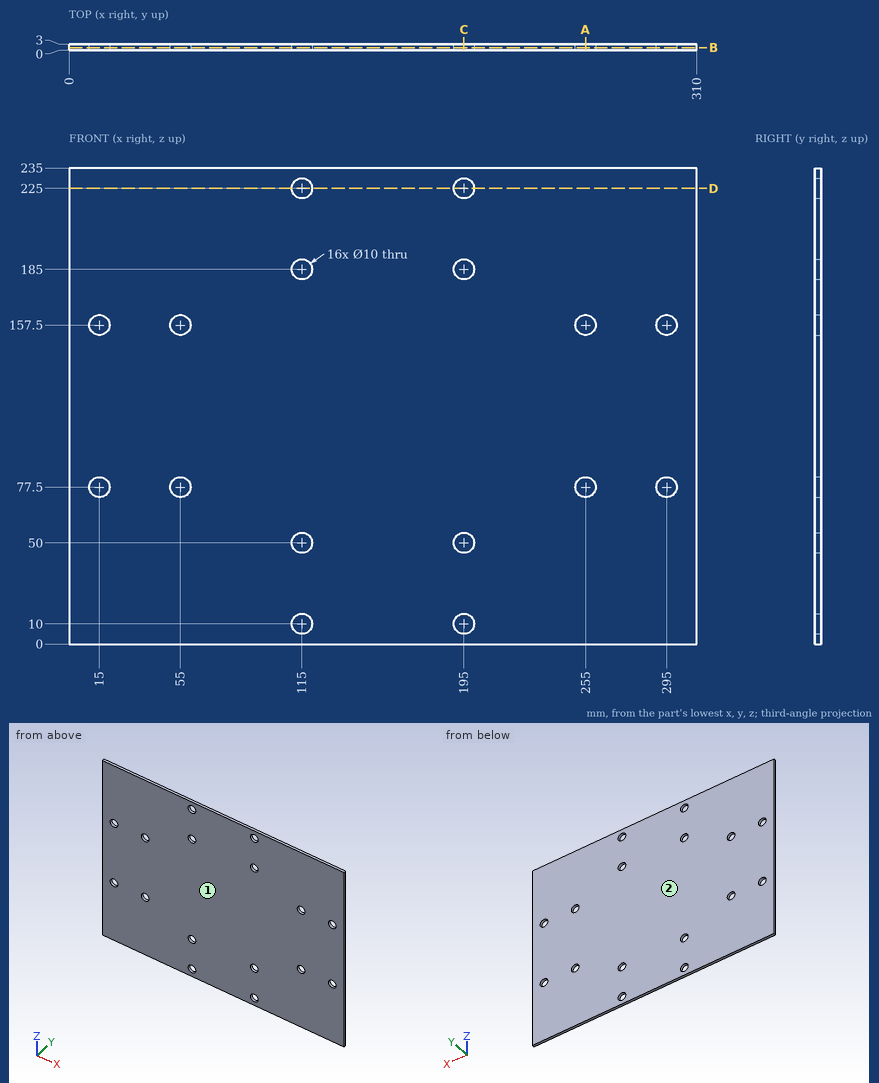
Study the drawing (mm; zero at the part's minimum x, y, z) and answer. Give positions to 0.01 mm unless a question says otherwise; leave off trailing zeros. Write each loop counter-clockwise with the first axis right and the second up, starting at its lowest first coordinate (ties: lowest second). Pieces come first, ordered by that corner, then holes.
Item 1: Section C-C, the plane x = 195 is taken. Write down the section's boundary in (y, z).
Item 2: Find the intervals of material crossed by line 1 along X through (y, z) = (2.4, 157.5); line 2 along Z through (x, y) = (195, 0.75); line 3 along X through (y, z) = (0.75, 50), in increasing order.
Item 3: Section D-D, the plane z = 225 is taken. Write down the section's boundary in (x, y).
Item 4: Determine the mould class of the marked faces 1 and 2 for opening direction Y: released by +Y, released by -Y, zero draft, split by the parting line, or undercut.
Item 5: Section A-A, the plane x = 255 is taken. Write down the section's boundary in (y, z).
Item 6: Section B-B, the plane y = 1.15 is taken. Count the separate pieces of the cut face and the enclosed holes in it, plus the area to 3 significant figures.
Completed:
1. outline: (0, 0) - (3, 0) - (3, 5) - (0, 5) - close; (0, 15) - (3, 15) - (3, 45) - (0, 45) - close; (0, 55) - (3, 55) - (3, 180) - (0, 180) - close; (0, 190) - (3, 190) - (3, 220) - (0, 220) - close; (0, 230) - (3, 230) - (3, 235) - (0, 235) - close
2. line 1: x = 0 to 10, 20 to 50, 60 to 250, 260 to 290, 300 to 310
2. line 2: z = 0 to 5, 15 to 45, 55 to 180, 190 to 220, 230 to 235
2. line 3: x = 0 to 110, 120 to 190, 200 to 310
3. outline: (0, 0) - (110, 0) - (110, 3) - (0, 3) - close; (120, 0) - (190, 0) - (190, 3) - (120, 3) - close; (200, 0) - (310, 0) - (310, 3) - (200, 3) - close
4. face 1: released by -Y
4. face 2: released by +Y
5. outline: (0, 0) - (3, 0) - (3, 72.5) - (0, 72.5) - close; (0, 82.5) - (3, 82.5) - (3, 152.5) - (0, 152.5) - close; (0, 162.5) - (3, 162.5) - (3, 235) - (0, 235) - close
6. separate pieces: 1
6. enclosed holes: 16
6. area: 71,600 mm2
